```python
from build123d import *

# Parameters (mm, degrees)
SKETCH1_R           = 5
BOSS_EXTRUDE1_DEPTH = 27.5
SKETCH11_R          = 2.5
CUT_EXTRUDE3_DEPTH  = 0.1
DOME2_FACE_RADIUS   = 2.5
DOME2_HEIGHT        = 2.5
CUT_EXTRUDE4_START  = -22.5
SKETCH12_R          = 5
SKETCH12_R_2        = 3.5
CUT_EXTRUDE4_DEPTH  = 22.5
CUT_EXTRUDE5_DEPTH  = 3
SKETCH14_W          = 3
SKETCH14_H          = 13.4
FILLET2_R           = 2
FILLET3_R           = 2


with BuildPart() as part:
    # Sketch1 → Boss-Extrude1 (new body)
    with BuildSketch(Plane(origin=(0, 0, 0), x_dir=(1, 0, 0), z_dir=(0, 1, 0))):
        with Locations(Location((0, 0, 0), (0, 0, 270))):
            Circle(SKETCH1_R)
    extrude(amount=BOSS_EXTRUDE1_DEPTH)

    # Sketch11 → Cut-Extrude3 (cut)
    with BuildSketch(Plane(origin=(0, 27.5, 0), x_dir=(1, 0, 0), z_dir=(0, 1, 0))):
        with Locations(Location((0, 0, 0), (0, 0, 270))):
            Circle(SKETCH11_R)
    extrude(amount=-CUT_EXTRUDE3_DEPTH, mode=Mode.SUBTRACT)

    # Dome2: an elliptical dome of height H over a round flat face of radius A is half a spheroid: the quarter ellipse of half axes A and H revolved about the face's axis
    with BuildSketch(Plane((0, 27.4, 0), x_dir=(0, 0, 1), z_dir=(1, 0, 0)), mode=Mode.PRIVATE) as dome2_quarter:
        Ellipse(DOME2_FACE_RADIUS, DOME2_HEIGHT)
        Rectangle(DOME2_FACE_RADIUS, DOME2_HEIGHT, align=(Align.MIN, Align.MIN), mode=Mode.INTERSECT)
    revolve(dome2_quarter.sketch, axis=Axis((0, 27.4, 0), (0, -1, 0)), mode=Mode.SUBTRACT)

    # Sketch12 → Cut-Extrude4 (cut)
    with BuildSketch(Plane(origin=(0, 27.5, 0), x_dir=(1, 0, 0), z_dir=(0, 1, 0)).offset(CUT_EXTRUDE4_START)):
        with Locations(Location((0, 0, 0), (0, 0, 270))):
            Circle(SKETCH12_R)
        with Locations(Location((0, 0, 0), (0, 0, 270))):
            Circle(SKETCH12_R_2, mode=Mode.SUBTRACT)
    extrude(amount=CUT_EXTRUDE4_DEPTH, mode=Mode.SUBTRACT)

    # Sketch2 → Cut-Extrude5 (cut)
    with BuildSketch(Plane.XZ):
        Polygon((-2.054262095, 3.480422471), (-4.041265323, -0.038831925), (-1.987003228, -3.519254396), (2.054262095, -3.480422471), (4.041265323, 0.038831925), (1.987003228, 3.519254396), align=None)
    extrude(amount=-CUT_EXTRUDE5_DEPTH, mode=Mode.SUBTRACT)

    # Sketch14 → Cut-Revolve1 (revolve, cut)
    with BuildSketch(Plane.XY, mode=Mode.PRIVATE) as cut_revolve1_sk:
        with Locations((3.5, 11.7)):
            Rectangle(SKETCH14_W, SKETCH14_H)
    revolve(cut_revolve1_sk.sketch.rotate(Axis((0, 0, 0), (0, 1, 0)), 270), axis=Axis((0, 0, 0), (0, 1, 0)), mode=Mode.SUBTRACT)

    # Fillet2
    fillet2_edges = [part.edges().sort_by_distance(p)[0] for p in [
        (0, 5, -2),
    ]]
    fillet(fillet2_edges, radius=FILLET2_R)

    # Fillet3
    # the kernel refuses this fillet: 2 mm, written as the material it adds along each edge
    with BuildSketch(Plane(origin=(0, 18.4, 0), x_dir=(0, 0, 1), z_dir=(-1, 0, 0))) as fillet3_piece_1:
        with BuildLine():
            CenterArc((4, -1.936491673), FILLET3_R, 104.477512186, 75.522487814)
            Line((3.5, 0), (3.49, 0.038729833))
            ThreePointArc((3.49, 0.038729833), (2.75, 0.04), (2, 0.04))
            Line((2, 0.04), (1.96, 0))
            Line((1.96, 0), (1.96, -1.936491673))
            Line((1.96, -1.936491673), (2, -1.936491673))
        make_face()
    revolve(axis=Axis((0, 18.4, 0), (0, 1, 0)))


solid = part.part
```
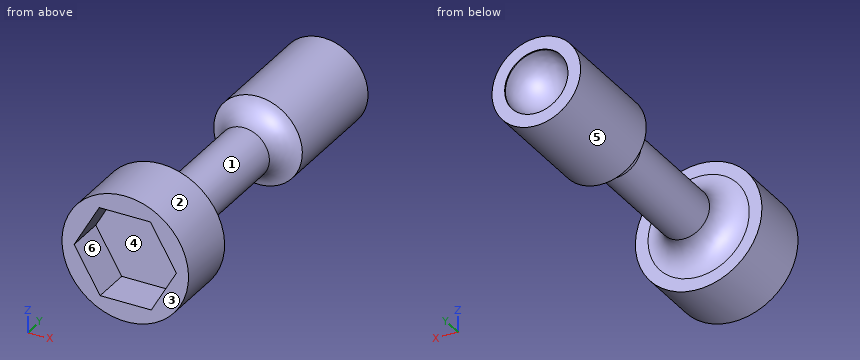
Can you work these out from the model? Positions are in its coordinate system, mm. Face numbers are marked on the shaded views. A direction names the side the tool comes from. Coordinates: 2 decimals unless noted, no trailing zeros. Loops run counter-clockwise (first coordinate to the right, second up) from the corner with the lowest first, then second, coordinate; pieces in that order, holes last.
Item 1: If we mould it in two halves opening along Z, with no side actions, what happens to the marked faces 3, 4, 5 and 6? For each: released by +Z, released by -Z, zero draft, split by the parting line, or undercut.
Answers below:
face 3: zero draft
face 4: undercut
face 5: split by the parting line
face 6: undercut
Item 2: I'm going to push flat-ended pins straight in: pin 1 (3 mm diameter, centred on x = 3, y = 24.5, fed in from +Z); pin 2 (4 mm diameter, centred on x = 0, y = 24, fed in from +Z); pin 3 (2 mm diameter, centred on x = 1.5, y = 17, fed in from -Z); pin 4 (6 mm diameter, centred on x = 0, z = 0, fed in from +Y). Where does each tip first touch, or does it pass through?
Answers below:
pin 1: stops at z = 3.16
pin 2: stops at z = 3.5
pin 3: stops at z = -2.38
pin 4: stops at y = 27.5
Item 3: Suppose I cut it at A-A (y = 22.75). Please give me the cut outline in (x, z).
Answers below:
outline: circle Ø7 at (0, 0)
Item 4: Please list where these lines run through material, in increasing order: L1, parallel to X at y = 27.4, z = 0; L2, parallel to Y at x = 4.75, z = 0.25; L3, parallel to X at y = 1.5, z = 2.75.
Answers below:
L1: x = -3.5 to -2.5, 2.5 to 3.5
L2: y = 0 to 5
L3: x = -4.18 to -2.47, 2.44 to 4.18
Item 5: Which directions (+Z, -Z, +X, -X, +Y, -Y) give clear straight access to the entire face, cutting with the end or side of a thin tool? Please do the marked faces 1 and 2.
Answers below:
face 1: none
face 2: +Y, -Y
Item 6: Suppose I cut it at B-B (y = 17). Please give me the cut outline in (x, z), then the cut area to 3 significant figures.
Answers below:
outline: circle Ø4.15 at (0, 0)
area: 13.5 mm2
